Check sheet for the drawn part. Datum: minimum x, y, z corner. Units: mm. Round coordinates to 2 decimals unless told otherwise and drop trailing zeros. Order: outer loops, then holes, each group sorted by start corner. A loop starts at its lowest first (then second) coordinate and runs counter-clockwise, first axis right, second up.
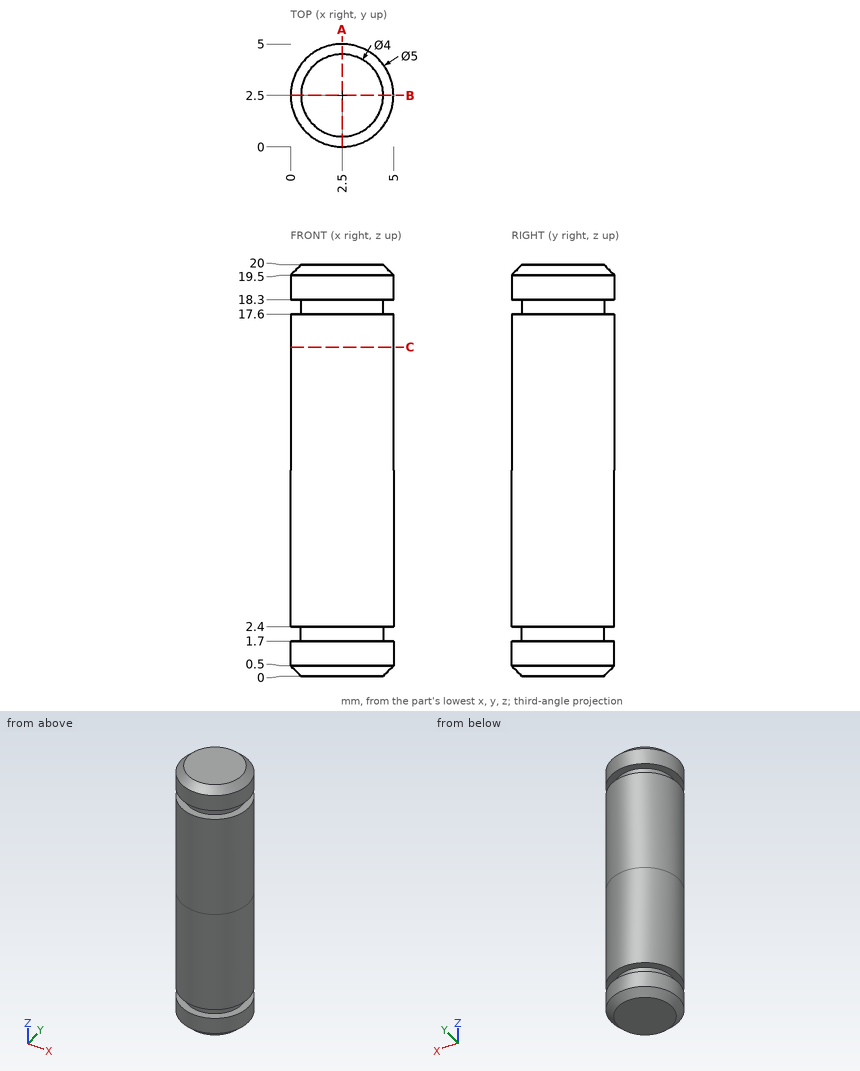
(1) Depth check by flat-ended pin: P1, Ø3, axis at x = 2.5, y = 4.5, coming from the -Z side. Enter the tip coordinate at first touch or a pass-through.
Returned:
P1: stops at z = 0
(2) Sectioned sample at C-C, the plane z = 16. Record the cut outline in (x, y).
Returned:
outline: circle Ø5 at (2.5, 2.5)
(3) Sectioned sample at A-A, the plane x = 2.5. Record the cut outline in (y, z), and give its area (3 significant figures).
Returned:
outline: (0, 0.5) - (0.5, 0) - (4.5, 0) - (5, 0.5) - (5, 1.7) - (4.5, 1.7) - (4.5, 2.4) - (5, 2.4) - (5, 17.6) - (4.5, 17.6) - (4.5, 18.3) - (5, 18.3) - (5, 19.5) - (4.5, 20) - (0.5, 20) - (0, 19.5) - (0, 18.3) - (0.5, 18.3) - (0.5, 17.6) - (0, 17.6) - (0, 2.4) - (0.5, 2.4) - (0.5, 1.7) - (0, 1.7) - close
area: 98.1 mm2
(4) Material ranges on line 1 (Z direction, x = 4.2, y = 3.8); line 2 (Z direction, x = 4.05, y = 1.2); line 3 (Y direction, x = 1, z = 7.5), recorded low to high.
Returned:
line 1: z = 0.14 to 1.7, 2.4 to 17.6, 18.3 to 19.86
line 2: z = 0.02 to 1.7, 2.4 to 17.6, 18.3 to 19.98
line 3: y = 0.5 to 4.5
